The listing builds one solid part. Answer for the finished solid, in the listing's coordinates (mm). A direction names the side the tool comes from. Coordinates: 2 decimals unless noted, no trailing zeros. Write each loop counter-clockwise with the first axis right and the second up, starting at its lowest first coordinate (ties: lowest second). Pieces come first, ordered by that corner, then holes.
Solid Edge part; units mm, degrees
sketch "Sketch1" plane through (0, 0, 0) normal (0, 0, 1) x (1, 0, 0)
  line L0 (6.75, -11.5) -> (-6.75, -11.5)
  line L1 (-6.75, -11.5) -> (-6.75, -17.9)
  line L2 (-6.75, -17.9) -> (6.75, -17.9)
  line L3 (6.75, -17.9) -> (6.75, -11.5)
  line L4 (0, -20.9) -> (9.5, -20.9)
  line L5 (9.5, -20.9) -> (9.5, -8.9)
  line L6 (9.5, -8.9) -> (6.15, 0)
  arc A0 (3, 5.3687) -> (6.15, 0) centre (0, 0) cw
  line L7 (3, 15) -> (3, 5.3687)
  line L8 (1, 15) -> (3, 15)
  line L9 (1, 4.0277) -> (1, 15)
  line L10 (-1, 15) -> (-1, 4.0277)
  line L11 (-1, 15) -> (-3, 15)
  line L12 (-3, 15) -> (-3, 5.3687)
  line L13 (-9.5, -8.9) -> (-6.15, 0)
  line L14 (-9.5, -20.9) -> (-9.5, -8.9)
  line L15 (0, -20.9) -> (-9.5, -20.9)
  arc A1 (1, 4.0277) -> (-1, 4.0277) centre (0, 0) cw
  arc A2 (-3, 5.3687) -> (-6.15, 0) centre (0, 0) ccw
extrude "Protrusion1" add sketch "Sketch1" along normal blind 10
fillet "Round_1" radius 2 8 edges at (-9.5, -20.9, 5) (9.5, -20.9, 5) (9.5, -8.9, 5) (-9.5, -8.9, 5) (6.15, 0, 5) (-6.15, 0, 5) (-3, 15, 5) (3, 15, 5)
sketch "Sketch2" plane through (3, 9.1843, 5) normal (1, 0, 0) x (0, 1, 0)
  circle A0 centre (0, 0) radius 1.65
extrude "ExtrudedCutout_1" cut sketch "Sketch2" against normal blind 6
sketch "Sketch3" plane through (-3, 9.1843, 5) normal (-1, 0, 0) x (0, -1, 0)
  line L0 (3, 1.7321) -> (0, 3.4641)
  line L1 (0, 3.4641) -> (-3, 1.7321)
  line L2 (-3, 1.7321) -> (-3, -1.7321)
  line L3 (-3, -1.7321) -> (0, -3.4641)
  line L4 (0, -3.4641) -> (3, -1.7321)
  line L5 (3, -1.7321) -> (3, 1.7321)
extrude "ExtrudedCutout_2" cut sketch "Sketch3" against normal blind 1
1. Section A-A on x = 0 is taken. Give the vertices of the cut face in (y, z).
Results found:
outline: (-20.9, 0) - (-17.9, 0) - (-17.9, 10) - (-20.9, 10) - close; (-11.5, 0) - (-4.15, 0) - (-4.15, 10) - (-11.5, 10) - close
2. Section C-C on x = -5.5 is taken. Give the vertices of the cut face in (y, z).
Results found:
outline: (-20.9, 0) - (-17.9, 0) - (-17.9, 10) - (-20.9, 10) - close; (-11.5, 0) - (2.75, 0) - (2.75, 10) - (-11.5, 10) - close
3. For a pull along X with two mould halves and no side action, classify faces 1 (the flat face through (6.75, -15, 5)), 2 (the cylindrical face through (-2.4, 14.43, 5.07)), 3 (the cylindrical face through (2.43, 14.4, 5.07)) as pulls with the +X half, pulls with the -X half, needs draft (parallel to the pull), parting line crosses it, or undercut.
Results found:
face 1: undercut
face 2: pulls with the -X half
face 3: pulls with the +X half
4. A tool of negligible diameter and unlimited length cuts with its end or side. For faces 4 (the flat face through (-2.507, 7.663, 7.586)), 5 (the flat face through (0, -11.5, 5)), 6 (the flat face through (-1, 11, 4)), from which of +Z, -Z, +X, -X, +Y, -Y can it reach the whole face along a straight path? Write none if from no direction.
Results found:
face 4: -X
face 5: +Z, -Z
face 6: +Z, -Z, +Y
5. Section B-B on z = 5 is taken. State how many separate pieces and enclosed holes the cut face has, then the cut area to 3 significant figures.
Results found:
separate pieces: 3
enclosed holes: 1
area: 300 mm2
6. Flat-ended cylindrical pins translate along their axes: P1, Ø4, axis at y = 11.5, z = 9, coming from the +X side; P2, Ø6, axis at y = 7.5, z = 8.5, coming from the -X side; P3, Ø5, axis at y = 10, z = 5.5, coming from the -X side. Find the tip coordinate at first contact, or state that the pin passes through.
Results found:
P1: stops at x = 3
P2: stops at x = -4.19
P3: stops at x = -3
7. Find the intervals of material crossed by L1, parallel to Y at x = 0, z = 7.25; L2, parallel to Y at x = -3.5, z = 1; L3, parallel to Y at x = 2.5, z = 8.5, in increasing order.
Results found:
L1: y = -20.9 to -17.9, -11.5 to -4.15
L2: y = -20.9 to -17.9, -11.5 to -2.23, 2.23 to 5.06
L3: y = -20.9 to -17.9, -11.5 to -3.31, 3.31 to 14.32
